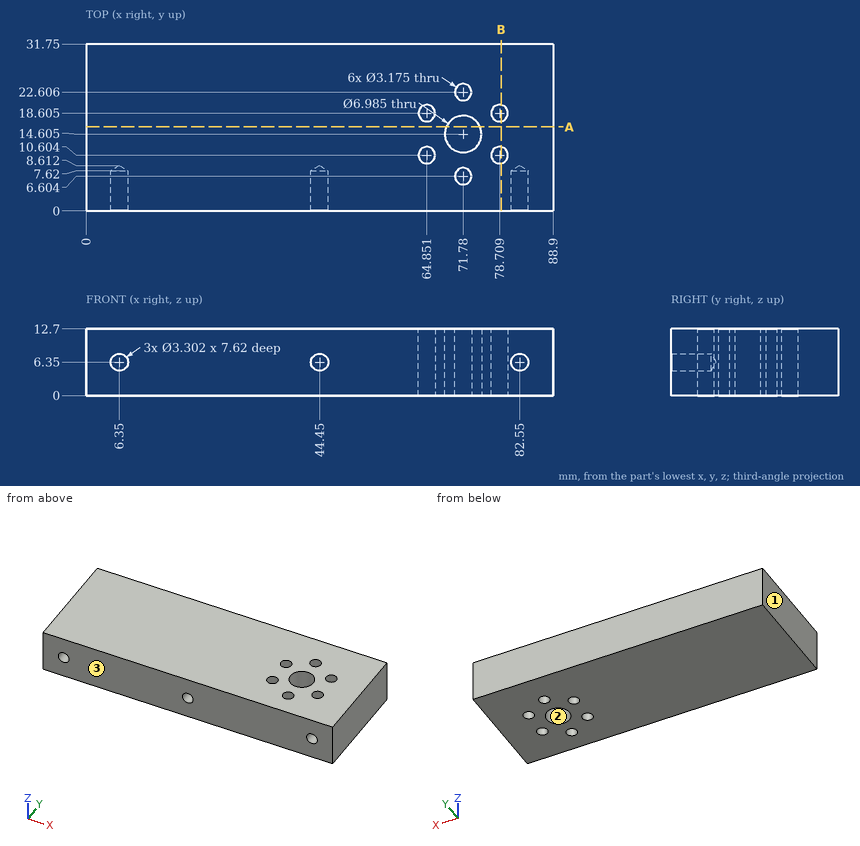
Here's the drawing with two shaded views (mm, measured from the low corner). I have some questions. Coordinates: 2 decimals unless noted, no trailing zeros. Order: outer loops, then holes, each group sorted by start corner. A loop starts at its lowest first (then second) coordinate and runs counter-clockwise, first axis right, second up. Notation, with made-up numbers: (81.25, 12) - (136.25, 12) arc R19 ccw to (136.25, 46) - close; hole circle Ø1 at (43, -18). An arc over 180 degrees is marked (long way). Answer in a Markdown table with one row per item. Add a question column.
(1) If we section it at A-A, the plane y = 16: Please give me the cut outline in (x, z), then the cut area to 3 significant figures.
(2) I need wall thicknesses on L1, parallel to X at y = 10.5, z = 0.75 (1 decimal); L2, parallel to X at y = 6, z = 6.35; L3, parallel to X at y = 22.5, z = 10 (1 decimal). Which ranges of each line are inside material? Lowest first, please.
(3) If we mould it in two halves opening along Y, with no side actions, what happens to the marked faces 1, 2 and 3? For each: released by +Y, released by -Y, zero draft, split by the parting line, or undercut.
(4) If we section it at B-B, the plane x = 79: State how many separate pieces and enclosed holes the cut face has, then the cut area to 3 significant figures.
(5) Will this pin go through, and if not, where does the flat tip stop? pin 1 (2 mm diameter, centred on x = 82.55, z = 6.35, fed in from -Y).
Results are:
| question | item | result |
|---|---|---|
| 1 | outline | (0, 0) - (68.58, 0) - (68.58, 12.7) - (0, 12.7) - close; (74.98, 0) - (88.9, 0) - (88.9, 12.7) - (74.98, 12.7) - close |
| 1 | area | 1,050 mm2 |
| 2 | L1 | x = 0 to 63.3, 66.4 to 77.1, 80.3 to 88.9 |
| 2 | L2 | x = 0 to 4.7, 8 to 42.8, 46.1 to 70.31, 73.25 to 80.9, 84.2 to 88.9 |
| 2 | L3 | x = 0 to 70.2, 73.4 to 88.9 |
| 3 | face 1 | zero draft |
| 3 | face 2 | undercut |
| 3 | face 3 | released by -Y |
| 4 | separate pieces | 3 |
| 4 | enclosed holes | 0 |
| 4 | area | 324 mm2 |
| 5 | pin 1 | stops at y = 8.01 |
